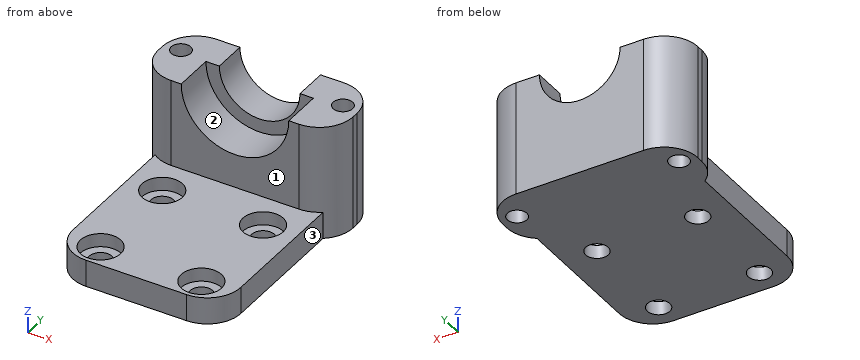
```python
from build123d import *

# Parameters (mm, degrees)
F0_W      = 25
F0_H      = 35
F1_DEPTH  = 4
F2_R      = 1.675
F3_DEPTH  = 25
F4_W      = 25
F4_H      = 11
F5_DEPTH  = 13
F7_DEPTH  = 6
F8_R      = 8
F9_DEPTH  = 6
F2_R_2    = 3
F10_DEPTH = 2
F11_R     = 5
F13_DEPTH = 2
F14_W     = 11
F14_H     = 17
F15_DEPTH = 2
F16_R     = 1.45
F17_DEPTH = 25
F18_R     = 5


with BuildPart() as f1:
    # F0 (on Top) → F1 (new body)
    with BuildSketch(Plane.XY):
        with Locations((12.5, 17.5)):
            Rectangle(F0_W, F0_H)
    extrude(amount=F1_DEPTH)

    # F2 (on face) → F3 (cut)
    with BuildSketch(Plane.XY.offset(4)):
        with BuildLine():
            ThreePointArc((3.325, 18.5605346784), (5, 16.8855346784), (6.675, 18.5605346784))
            ThreePointArc((6.675, 18.5605346784), (5, 20.2355346784), (3.325, 18.5605346784))
        make_face()
        with Locations((20, 18.5605346784)):
            Circle(F2_R)
        with Locations((20, 3.5605346784)):
            Circle(F2_R)
        with Locations((5, 3.5605346784)):
            Circle(F2_R)
    extrude(amount=-F3_DEPTH, mode=Mode.SUBTRACT)

    # F4 (on face) → F5 (join)
    with BuildSketch(Plane.XY.offset(4)):
        with Locations((12.5, 29.5)):
            Rectangle(F4_W, F4_H)
    extrude(amount=F5_DEPTH)

    # F6 (on face) → F7 (cut)
    with BuildSketch(Plane(origin=(0, 35, 0), x_dir=(-1, 0, 0), z_dir=(0, 1, 0))):
        with BuildLine():
            ThreePointArc((-18.5, 17), (-12.5, 11), (-6.5, 17))
            Line((-6.5, 17), (-18.5, 17))
        make_face()
    extrude(amount=-F7_DEPTH, mode=Mode.SUBTRACT)

    # F8 (on face) → F9 (cut)
    with BuildSketch(Plane.XZ.offset(-24)):
        with Locations((12.5, 17)):
            Circle(F8_R)
    extrude(amount=-F9_DEPTH, mode=Mode.SUBTRACT)

    # F2 (on face) → F10 (cut)
    with BuildSketch(Plane.XY.offset(4)):
        with BuildLine():
            ThreePointArc((8, 18.5605346784), (5, 21.5605346784), (2, 18.5605346784))
            ThreePointArc((2, 18.5605346784), (5, 15.5605346784), (8, 18.5605346784))
        make_face()
        with BuildLine():
            ThreePointArc((3.325, 18.5605346784), (5, 20.2355346784), (6.675, 18.5605346784))
            ThreePointArc((6.675, 18.5605346784), (5, 16.8855346784), (3.325, 18.5605346784))
        make_face(mode=Mode.SUBTRACT)
        with Locations((20, 18.5605346784)):
            Circle(F2_R_2)
        with Locations((20, 18.5605346784)):
            Circle(F2_R, mode=Mode.SUBTRACT)
        with Locations((20, 3.5605346784)):
            Circle(F2_R_2)
        with Locations((20, 3.5605346784)):
            Circle(F2_R, mode=Mode.SUBTRACT)
        with Locations((5, 3.5605346784)):
            Circle(F2_R_2)
        with Locations((5, 3.5605346784)):
            Circle(F2_R, mode=Mode.SUBTRACT)
    extrude(amount=-F10_DEPTH, mode=Mode.SUBTRACT)

    # F11
    f11_edges = [f1.edges().sort_by_distance(p)[0] for p in [
        (0, 0, 2),
        (25, 0, 2),
    ]]
    fillet(f11_edges, radius=F11_R)

    # F12 (on face) + F5_face3 (on face) → F13 (join)
    with BuildSketch(Plane(origin=(0, 0, 0), x_dir=(0, -1, 0), z_dir=(-1, 0, 0))):
        Polygon((-35, 17), (-35, 0), (-24, 0), (-24, 4), (-24, 17), align=None)
    with BuildSketch(Plane(origin=(25, 25.1653992395, 6.6216730038), x_dir=(0, 1, 0), z_dir=(1, 0, 0))):
        Polygon((-1.1653992395, -2.6216730038), (-20.1653992395, -2.6216730038), (-20.1653992395, -6.6216730038), (9.8346007605, -6.6216730038), (9.8346007605, 10.3783269962), (-1.1653992395, 10.3783269962), align=None)
    extrude(amount=F13_DEPTH, dir=(-1, 0, 0))

    # F14 (on face) → F15 (join)
    with BuildSketch(Plane.YZ.offset(25)):
        with Locations((29.5, 8.5)):
            Rectangle(F14_W, F14_H)
    extrude(amount=F15_DEPTH)

    # F16 (on face) → F17 (cut)
    with BuildSketch(Plane.XY.offset(17)):
        with Locations((0.45, 30.55)):
            Circle(F16_R)
        with Locations((24.55, 30.55)):
            Circle(F16_R)
    extrude(amount=-F17_DEPTH, mode=Mode.SUBTRACT)

    # F18
    f18_edges = [f1.edges().sort_by_distance(p)[0] for p in [
        (-2, 24, 8.5),
        (-2, 35, 8.5),
        (27, 35, 8.5),
        (27, 24, 8.5),
    ]]
    fillet(f18_edges, radius=F18_R)


solid = f1.part
```
Part model, mm, in its own coordinate system. Face numbers are marked on the shaded views. A direction names the side the tool comes from. Coordinates: 2 decimals unless noted, no trailing zeros. Loops run counter-clockwise (first coordinate to the right, second up) from the corner with the lowest first, then second, coordinate; pieces in that order, holes last. Notation, with made-up numbers: (69.25, 14) - (80.25, 14) arc R4 ccw to (80.25, 18) - close; hole circle Ø11 at (64.25, 62). An arc over 180 degrees is marked (long way). Write item = value, one per line. Start each with the question number.
Item 1: Cut at C-C, the plane x = 0.45. Give the cut face in (y, z), and give its area (3 significant figures).
Item 2: Wall check: L1, parallel to Y at x = 20, z = 1.1; L2, parallel to Y at x = 5, z = 3.35; L3, parallel to X at y = 4, z = 3.75. Give the ranges that are in metal, low to high. Write a range as from..to.
Item 3: Cut at A-A, the plane z = 15. Give the cut face in (x, y), and give its area (3 significant figures).
Item 4: Cut at B-B, the plane y = 30.55. Give the cut face in (x, z), and give its area (3 significant figures).
Item 5: Cut at D-D, the plane z = 5. Give the cut face in (x, y), and give its area (3 significant figures).
Item 6: Flat gauge pins, fed straight in: pin 1 Ø7.5 at (x, y) = (18.5, 15.5) entering from +Z; pin 2 Ø5 at (x, y) = (13.5, 22.5) entering from +Z; pin 3 Ø8 at (x, y) = (11, 23) entering from +Z; pin 4 Ø2.5 at (x, y) = (5, 3.56) entering from -Z. Where does each tip first touch, or does it go through?
Item 7: 3-axis set-ups, long thin cutter, end or side, ignore diameter. For the marked faces 1, 2 and 3: which of +Z, -Z, +X, -X, +Y, -Y reach the whole face in a straight line?
The answers:
q1.outline = (2.93, 0) - (29.1, 0) - (29.1, 17) - (24.7, 17) - (24.7, 4) - (2.93, 4) - close; (32, 0) - (34.3, 0) - (34.3, 17) - (32, 17) - close
q1.area = 201 mm2
q2.L1 = 0..1.89, 5.24..16.89, 20.24..35
q2.L2 = 0..0.56, 6.56..15.56, 21.56..35
q2.L3 = 0.1..2.03, 7.97..17.03, 22.97..24.9
q3.outline = (-2, 29) arc R5 ccw to (3, 24) - (4.75, 24) - (4.75, 30) - (6.84, 30) - (6.84, 35) - (3, 35) arc R5 ccw to (-2, 30) - close; (18.16, 30) - (20.25, 30) - (20.25, 24) - (22, 24) arc R5 ccw to (27, 29) - (27, 30) arc R5 ccw to (22, 35) - (18.16, 35) - close; hole circle Ø2.9 at (0.45, 30.55); hole circle Ø2.9 at (24.55, 30.55)
q3.area = 135 mm2
q4.outline = (-1.97, 0) - (-1, 0) - (-1, 17) - (-1.97, 17) - close; (1.9, 0) - (23.1, 0) - (23.1, 17) - (18.5, 17) arc R6 cw to (6.5, 17) - (1.9, 17) - close; (26, 0) - (26.97, 0) - (26.97, 17) - (26, 17) - close
q4.area = 337 mm2
q5.outline = (-2, 29) arc R5 ccw to (3, 24) - (22, 24) arc R5 ccw to (27, 29) - (27, 30) arc R5 ccw to (22, 35) - (3, 35) arc R5 ccw to (-2, 30) - close; hole circle Ø2.9 at (0.45, 30.55); hole circle Ø2.9 at (24.55, 30.55)
q5.area = 284 mm2
q6.pin_1 = 4
q6.pin_2 = 9.58
q6.pin_3 = 11.07
q6.pin_4 = through
q7.face_1 = +Z, +X, -X, -Y
q7.face_2 = +Z, -Y
q7.face_3 = +Z, -Z, +X, -Y
